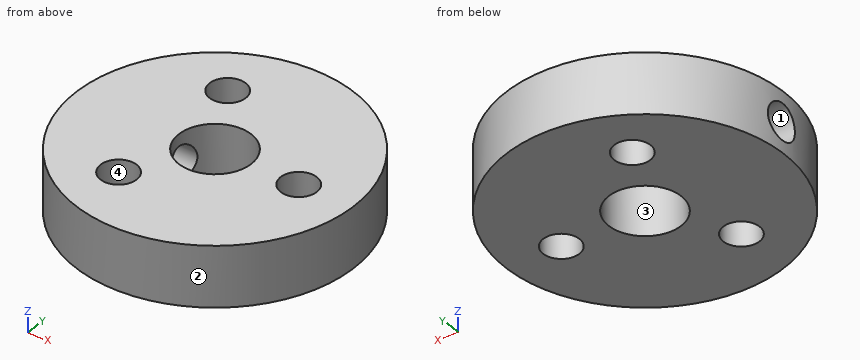
Autodesk Inventor part; units mm, degrees
ref_plane "YZ Plane" through (0, 0, 0) normal (1, 0, 0) x (0, 1, 0)
ref_plane "XZ Plane" through (0, 0, 0) normal (0, 1, 0) x (-1, 0, 0)
ref_plane "XY Plane" through (0, 0, 0) normal (0, 0, 1) x (1, 0, 0)
sketch "Sketch3" plane through (0, 0, 0) normal (0, 0, 1) x (1, 0, 0)
  circle A0 centre (0, 0) radius 11.5
  circle A1 centre (0, 0) radius 3
  circle A2 centre (7, 0) radius 1.5
  circle A3 centre (3.5, 6.0622) radius 1.5
  circle A4 centre (-3.5, 6.0622) radius 1.5
  circle A5 centre (-7, 0) radius 1.5
  circle A6 centre (-3.5, -6.0622) radius 1.5
  circle A7 centre (3.5, -6.0622) radius 1.5
  dimension "d0" = 23
  dimension "d1" = 6
  dimension "d4" = 3
  dimension "d5" = 7
  dimension "d12" = 360
extrude "Extrusion1" add sketch "Sketch3" along normal blind 5 contours A0 | A3 | A5 | A7
sketch "Sketch4" plane through (0, 0, 0) normal (1, 0, 0) x (0, 1, 0)
  line L0 (-11.5, 0) -> (11.5, 0)
  line L1 (-3, 5) -> (3, 5)
  line L2 (3, 0) -> (-3, 0)
  circle A0 centre (0, 2.5) radius 1.5
  line L3 (3, 0) -> (3, 5)
  point P0 (0, 0)
  point P1 (0, 0)
  point P2 (3, 2.5)
  dimension "d14" = 3
extrude "Extrusion2" cut sketch "Sketch4" against normal through all
thread "Thread1"
thread "Thread2"
thread "Thread3"
thread "Thread4"
equation "\"d15\" = d14"
properties part number "6mm Mounting Hub, thin" material "Aluminum 6061"
The model under review builds one solid part; all positions refer to its coordinate system, in mm. Face numbers are marked on the shaded views. Give positions to 0.01 mm unless a question says otherwise; leave off trailing zeros. Loops run counter-clockwise (first coordinate to the right, second up) from the corner with the lowest first, then second, coordinate; pieces in that order, holes last. Notation, with made-up numbers: (6, 53) -> (22, 53) arc R27 ccw to (22, 71) -> close; hole circle Ø6 at (-21, 0). An arc over 180 degrees is marked (long way). Answer as a JSON object with one key per item and string values. Group by question number.
Q1. Take a section at C-C (x = -3.5). Write out the cut boundary in (y, z).
Q2. Take a section at D-D (z = 3.65). Write out the cut boundary in (x, y).
Q3. Take a section at B-B (x = 0). Write out the cut boundary in (y, z), plus the area to 3 significant figures.
Q4. Take a section at A-A (y = 0). Write out the cut boundary in (x, z), plus the area to 3 significant figures.
Q5. Wall thickness on line 1 along Y through (x, z) = (-3.5, 2.6); line 2 along Y through (x, z) = (-3.5, 1.9); line 3 along Y through (x, z) = (-4.5, 4.5): over which ranges is each line inside the solid? List them lowest first.
Q6. Draft analysis for pull direction X (two halves, no side actions). For the marked faces 1, 2, 3 and 4, state which applies: pulls with the +X half, pulls with the -X half, needs draft (parallel to the pull), parting line crosses it, or undercut.
Q7. Insertion check: pin 1 (3 mm diameter, centred on y = 7.5, z = 0.5, fed in from -X); pin 2 (2.5 mm diameter, centred on x = 7, y = 0, fed in from -Z); pin 3 (1 mm diameter, centred on x = 5, z = 2.5, fed in from -Y); pin 4 (1 mm diameter, centred on y = -7.5, z = 3.5, fed in from -X). Each pin has a flat end and moves straight along its axis. Give the tip position at first contact, or say it passes through.
Answer below:
{
 "1": {"outline": "(-10.95, 0) -> (-7.56, 0) -> (-7.56, 5) -> (-10.95, 5) -> close; (-4.56, 0) -> (4.56, 0) -> (4.56, 5) -> (-4.56, 5) -> close; (7.56, 0) -> (10.95, 0) -> (10.95, 5) -> (7.56, 5) -> close; hole circle Ø3 at (0, 2.5)"},
 "2": {"outline": "(-11.46, -0.96) arc R11.5 ccw (long way) to (-11.46, 0.96) -> (-2.84, 0.96) arc R3 cw (long way) to (-2.84, -0.96) -> close; hole circle Ø3 at (-3.5, -6.06); hole circle Ø3 at (-3.5, 6.06); hole circle Ø3 at (7, 0)"},
 "3": {"outline": "(-11.5, 0) -> (-3, 0) -> (-3, 5) -> (-11.5, 5) -> close; (3, 0) -> (11.5, 0) -> (11.5, 5) -> (3, 5) -> close", "area": "85.0 mm2"},
 "4": {"outline": "(-11.5, 0) -> (-3, 0) -> (-3, 1) -> (-11.5, 1) -> close; (-11.5, 4) -> (-3, 4) -> (-3, 5) -> (-11.5, 5) -> close; (3, 0) -> (5.5, 0) -> (5.5, 5) -> (3, 5) -> close; (8.5, 0) -> (11.5, 0) -> (11.5, 5) -> (8.5, 5) -> close", "area": "44.5 mm2"},
 "5": {"line 1": "y = -10.95 to -7.56, -4.56 to -1.5, 1.5 to 4.56, 7.56 to 10.95", "line 2": "y = -10.95 to -7.56, -4.56 to -1.37, 1.37 to 4.56, 7.56 to 10.95", "line 3": "y = -10.58 to -7.18, -4.94 to 4.94, 7.18 to 10.58"},
 "6": {"face 1": "needs draft", "face 2": "parting line crosses it", "face 3": "undercut", "face 4": "undercut"},
 "7": {"pin 1": "stops at x = -9.81", "pin 2": "passes through", "pin 3": "stops at y = -10.58", "pin 4": "stops at x = -9.12"}
}
